from build123d import *

# Parameters (mm, degrees)
F0_W      = 53.975
F0_H      = 85.725
F1_DEPTH  = 1.5875
F3_W      = 53.5911135375
F3_H      = 29.5717269182
F4_DEPTH  = 1.5875
F2_W      = 53.975
F2_H      = 30.1625
F5_DEPTH  = 1.5875
F9_DEPTH  = 1.5875
F10_DEPTH = 1.5875


# Not quite as in the source:
# - the program builds the solid bodies; features that only make, move or delete a surface that nothing else refers to are left out


with BuildPart() as f1:
    # F0 (on Top) → F1 (new body)
    with BuildSketch(Plane.XY):
        Rectangle(F0_W, F0_H)
    extrude(amount=F1_DEPTH)

    # F3 (on face) → F4 (join)
    with BuildSketch(Plane.XY.offset(1.5875)):
        with Locations((0.1150835305, -27.1980315447)):
            Rectangle(F3_W, F3_H)
    extrude(amount=F4_DEPTH)

    # F2 (on face) → F5 (join)
    with BuildSketch(Plane.XY.offset(1.5875)):
        with Locations((0, 27.78125)):
            Rectangle(F2_W, F2_H)
    extrude(amount=F5_DEPTH)

    # F8 (on face) → F9 (join)
    with BuildSketch(Plane.XY.offset(1.5875)):
        with BuildLine():
            ThreePointArc((-3.175, -11.7439402944), (0, -12.1655562404), (3.175, -11.7439402944))
            Line((3.175, -11.7439402944), (3.175, 11.7439402944))
            ThreePointArc((3.175, 11.7439402944), (0, 12.1655562404), (-3.175, 11.7439402944))
            Line((-3.175, 11.7439402944), (-3.175, -11.7439402944))
        make_face()
    extrude(amount=F9_DEPTH)

    # F10 (add): a face of the model
    f10_faces = [f1.faces().sort_by_distance(p)[0] for p in [
        (0, 0, 3.175),
    ]]
    extrude(f10_faces, amount=F10_DEPTH)


solid = f1.part
Here's how the part is built. I have some questions about the finished solid (model axes, mm). A direction names the side the tool comes from. Coordinates: 2 decimals unless noted, no trailing zeros. Loops run counter-clockwise (first coordinate to the right, second up) from the corner with the lowest first, then second, coordinate; pieces in that order, holes last.
1. I need wall thicknesses on L1, parallel to Y at x = 5.5, z = 2.4; L2, parallel to X at y = -32, z = 2.7; L3, parallel to Z at x = -13, y = 9. Which ranges of each line are inside material? Lowest first, please.
2. Imagine slicing it at B-B, the plane y = -9. Please give me the cut outline in (x, z) (1 decimal).
3. For faces 4 (the flat face through (0, 12.7, 2)), 5 (the flat face through (0, -41.984, 2)), 6 (the cylindrical face through (-0.045, -12.165, 3.153)), which set-ups out of +Z, -Z, +X, -X, +Y, -Y let a thin tool reach every point of the face, with its end or its side?
4. If we mould it in two halves opening along Y, with no side actions, what happens to faces 1 (the flat face through (0, -12.412, 2)), 2 (the flat face through (0, -27, 3.175)), 3 (the flat face through (0, -42.862, 1))? For each: pulls with the +Y half, pulls with the -Y half, needs draft (parallel to the pull), parting line crosses it, or undercut.
5. Imagine slicing it at A-A, the plane x = 11. Please give me the cut outline in (y, z) (1 decimal), and give its area (3 significant figures).
6. Imagine slicing it at C-C, the plane z = 3.9. Please give me the cut outline in (x, y) (3 decimals), and give its area (3 significant figures).
7. For P1, Ø0.8, axis at x = -0.5, z = 2.5, coming from the -Y side; P2, Ø16, axis at x = -11.5, y = -19, coming from the +Z side (3 decimals); P3, Ø0.8, axis at y = -22, z = 2.5, coming from the -X side, each with a flat end and sliding along its axis, tell me the tip position at first contact or that it passes through.
Taken from the geometry:
1. L1: y = -41.98 to -12.41, 12.7 to 42.86
1. L2: x = -26.68 to 26.91
1. L3: z = 0 to 1.59
2. outline: (-27, 0) - (27, 0) - (27, 1.6) - (3.2, 1.6) - (3.2, 4.8) - (-3.2, 4.8) - (-3.2, 1.6) - (-27, 1.6) - close
3. face 4: +Z, +X, -X
3. face 5: +Z, +X, -X, -Y
3. face 6: +Z
4. face 1: undercut
4. face 2: needs draft
4. face 3: pulls with the -Y half
5. outline: (-42.9, 0) - (42.9, 0) - (42.9, 3.2) - (12.7, 3.2) - (12.7, 1.6) - (-12.4, 1.6) - (-12.4, 3.2) - (-42, 3.2) - (-42, 1.6) - (-42.9, 1.6) - close
5. area: 231 mm2
6. outline: (-3.175, -11.744) arc R12.166 ccw to (3.175, -11.744) - (3.175, 11.744) arc R12.166 ccw to (-3.175, 11.744) - close
6. area: 153 mm2
7. P1: stops at y = -41.98
7. P2: stops at z = 3.175
7. P3: stops at x = -26.68
